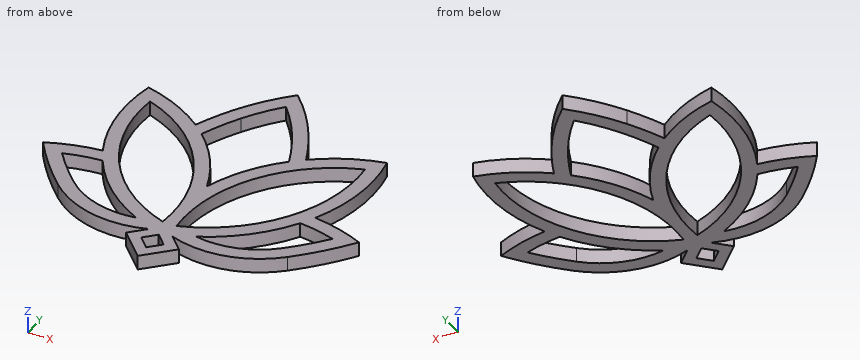
```python
from build123d import *

# Parameters (mm, degrees)
BOSS_EXTRUDE1_DEPTH = 1


with BuildPart() as part:
    # Sketch1 → Boss-Extrude1 (new body)
    with BuildSketch(Plane.XY):
        with BuildLine():
            Line((0, 0), (1.838477631, 1.838477631))
            Line((1.838477631, 1.838477631), (0.823678808, 2.853276454))
            ThreePointArc((0.823678808, 2.853276454), (4.623918861, 2.588642918), (8, 4.353276454))
            ThreePointArc((8, 4.353276454), (9.591924549, 6.024483983), (11, 7.853276454))
            ThreePointArc((11, 7.853276454), (9.237519313, 8.488345979), (7.4, 8.853276454))
            ThreePointArc((7.4, 8.853276454), (8.450856423, 12.419917717), (8.3, 16.135085474))
            ThreePointArc((8.3, 16.135085474), (5.960145608, 15.324834522), (3.85, 14.029183838))
            ThreePointArc((3.85, 14.029183838), (3.284007759, 15.28410345), (2.63, 16.495484604))
            ThreePointArc((2.63, 16.495484604), (1.429185762, 18.254368816), (0, 19.833310412))
            ThreePointArc((0, 19.833310412), (-1.429185762, 18.254368816), (-2.63, 16.495484604))
            ThreePointArc((-2.63, 16.495484604), (-3.284007759, 15.28410345), (-3.85, 14.029183838))
            ThreePointArc((-3.85, 14.029183838), (-5.960145608, 15.324834522), (-8.3, 16.135085474))
            ThreePointArc((-8.3, 16.135085474), (-8.450856423, 12.419917717), (-7.4, 8.853276454))
            ThreePointArc((-7.4, 8.853276454), (-9.237519313, 8.488345979), (-11, 7.853276454))
            ThreePointArc((-11, 7.853276454), (-9.591924549, 6.024483983), (-8, 4.353276454))
            ThreePointArc((-8, 4.353276454), (-4.623918861, 2.588642918), (-0.823678808, 2.853276454))
            Line((-0.823678808, 2.853276454), (-1.838477631, 1.838477631))
            Line((-1.838477631, 1.838477631), (0, 0))
        make_face()
        Polygon((0, 1.060660172), (0.777817459, 1.838477631), (0, 2.61629509), (-0.777817459, 1.838477631), align=None, mode=Mode.SUBTRACT)
        with BuildLine():
            ThreePointArc((1.767555689, 15.989332639), (2.460089794, 14.692656758), (3.046312622, 13.344578636))
            ThreePointArc((3.046312622, 13.344578636), (1.223262024, 11.152840308), (0, 8.577794598))
            ThreePointArc((0, 8.577794598), (-1.223262024, 11.152840308), (-3.046312622, 13.344578636))
            ThreePointArc((-3.046312622, 13.344578636), (-2.460089794, 14.692656758), (-1.767555689, 15.989332639))
            ThreePointArc((-1.767555689, 15.989332639), (-0.945525016, 17.238680092), (0, 18.397380194))
            ThreePointArc((0, 18.397380194), (0.945525016, 17.238680092), (1.767555689, 15.989332639))
        make_face(mode=Mode.SUBTRACT)
        with BuildLine():
            ThreePointArc((7.484522548, 14.86555012), (2.078927518, 10.634692843), (0.478972095, 3.959308692))
            ThreePointArc((0.478972095, 3.959308692), (5.884567125, 8.190165969), (7.484522548, 14.86555012))
        make_face(mode=Mode.SUBTRACT)
        with BuildLine():
            ThreePointArc((2.091646058, 3.542273843), (4.886787797, 3.684978553), (7.313103604, 5.080031806))
            ThreePointArc((7.313103604, 5.080031806), (8.408951023, 6.195914234), (9.418710619, 7.390259542))
            ThreePointArc((9.418710619, 7.390259542), (8.165419306, 7.717459739), (6.883314947, 7.901870952))
            ThreePointArc((6.883314947, 7.901870952), (4.803155716, 5.375111185), (2.091646058, 3.542273843))
        make_face(mode=Mode.SUBTRACT)
        with BuildLine():
            ThreePointArc((-6.883314947, 7.901870952), (-8.165419306, 7.717459739), (-9.418710619, 7.390259542))
            ThreePointArc((-9.418710619, 7.390259542), (-8.408951023, 6.195914234), (-7.313103604, 5.080031806))
            ThreePointArc((-7.313103604, 5.080031806), (-4.886787797, 3.684978553), (-2.091646058, 3.542273843))
            ThreePointArc((-2.091646058, 3.542273843), (-4.803155716, 5.375111185), (-6.883314947, 7.901870952))
        make_face(mode=Mode.SUBTRACT)
        with BuildLine():
            ThreePointArc((-7.484522548, 14.86555012), (-5.884567125, 8.190165969), (-0.478972095, 3.959308692))
            ThreePointArc((-0.478972095, 3.959308692), (-2.078927518, 10.634692843), (-7.484522548, 14.86555012))
        make_face(mode=Mode.SUBTRACT)
    extrude(amount=BOSS_EXTRUDE1_DEPTH)


solid = part.part
```
Check sheet for the modelled part. Datum: model origin and axes. Units: mm. Give positions to 0.01 mm unless a question says otherwise; leave off trailing zeros. Order: outer loops, then holes, each group sorted by start corner. A loop starts at its lowest first (then second) coordinate and runs counter-clockwise, first axis right, second up. Notation, with made-up numbers: (14.5, 24.25) -> (70.5, 24.25) arc R24 cw to (70.5, 56.25) -> close; hole circle Ø4 at (-23, -33). An arc over 180 degrees is marked (long way). Use CSV: the item, a comma, the result in double quotes. Start each with the question number.
1) Material ranges on line 1 (X direction, y = 13.5, z = 0.4); line 2 (X direction, y = 9, z = 0.1); line 3 (X direction, y = 7, z = 0.75), recorded low to high. Write a range as from..to.
2) Sectioned sample at D-D, the plane z = 0.4. Give the number of separate pieces and of enclosed holes in the cut face, plus the area to 3 significant figures.
3) Sectioned sample at C-C, the plane y = 12.75. Record the boundary of the cut face in (x, z).
4) Sectioned sample at A-A, the plane y = 7. Record the boundary of the cut face in (x, z).
5) Sectioned sample at B-B, the plane x = -5.75. Record the boundary of the cut face in (y, z).
Recorded:
1,line 1,"-8.53..-7.53, -4.81..-2.99, 2.99..4.81, 7.53..8.53"
1,line 2,"-7.47..-6.35, -1.22..-0.15, 0.15..1.22, 6.35..7.47"
1,line 3,"-10.38..-9.11, -6.28..-4.99, -0.62..0.62, 4.99..6.28, 9.11..10.38"
2,separate pieces,"1"
2,enclosed holes,"6"
2,area,"104 mm2"
3,outline,"(-8.49, 0) -> (-7.48, 0) -> (-7.48, 1) -> (-8.49, 1) -> close; (-3.88, 0) -> (-2.46, 0) -> (-2.46, 1) -> (-3.88, 1) -> close; (2.46, 0) -> (3.88, 0) -> (3.88, 1) -> (2.46, 1) -> close; (7.48, 0) -> (8.49, 0) -> (8.49, 1) -> (7.48, 1) -> close"
4,outline,"(-10.38, 0) -> (-9.11, 0) -> (-9.11, 1) -> (-10.38, 1) -> close; (-6.28, 0) -> (-4.99, 0) -> (-4.99, 1) -> (-6.28, 1) -> close; (-0.62, 0) -> (0.62, 0) -> (0.62, 1) -> (-0.62, 1) -> close; (4.99, 0) -> (6.28, 0) -> (6.28, 1) -> (4.99, 1) -> close; (9.11, 0) -> (10.38, 0) -> (10.38, 1) -> (9.11, 1) -> close"
5,outline,"(2.92, 0) -> (4.01, 0) -> (4.01, 1) -> (2.92, 1) -> close; (6.35, 0) -> (7.99, 0) -> (7.99, 1) -> (6.35, 1) -> close; (14.09, 0) -> (15.22, 0) -> (15.22, 1) -> (14.09, 1) -> close"
